Geometry check sheet. Reference: drawing and pictorial views, mm from the part's lowest x, y, z. A direction names the side the tool comes from. Round coordinates to 2 decimals unless told otherwise and drop trailing zeros. Write each loop counter-clockwise with the first axis right and the second up, starting at its lowest first coordinate (ties: lowest second). Pieces come first, ordered by that corner, then holes. Notation, with made-up numbers: M 69,14.5 L 96,14.5 A30 cw 96,53.5 Z; hole C 86.5,-40 d10. An arc over 180 degrees is marked long. Answer in a Markdown table with one row per item.
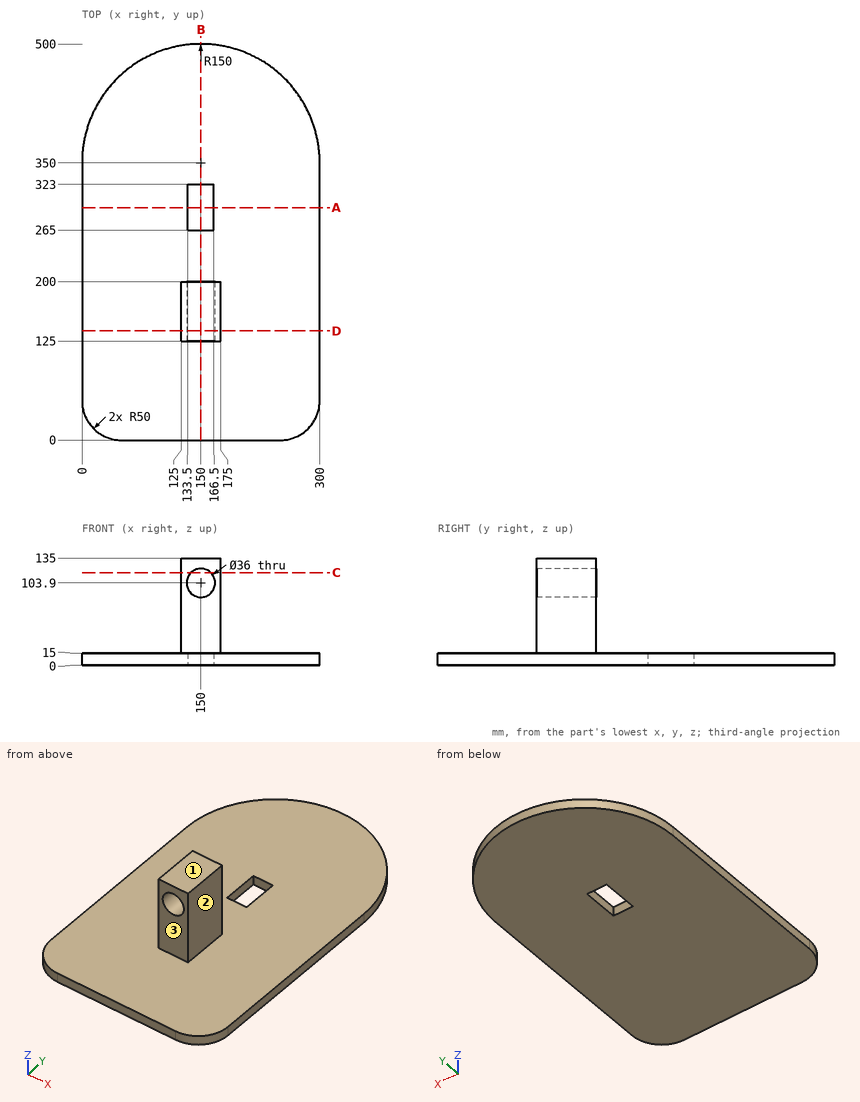
1. Section check C-C, the plane z = 117. Record the cut outline in (x, y).
Found:
| item | result |
|---|---|
| outline | M 125,125 L 137.66,125 L 137.66,200 L 125,200 Z; M 162.34,125 L 175,125 L 175,200 L 162.34,200 Z |
2. Section check B-B, the plane x = 150. Record the cut outline in (y, z).
Found:
| item | result |
|---|---|
| outline | M 0,0 L 265,0 L 265,15 L 200,15 L 200,85.9 L 125,85.9 L 125,15 L 0,15 Z; M 125,121.9 L 200,121.9 L 200,135 L 125,135 Z; M 323,0 L 500,0 L 500,15 L 323,15 Z |
3. Scan lines: L1, parallel to X at y = 154, z = 103; L2, parallel to Z at x = 150, y = 161; L3, parallel to Z at x = 220, y = 122.5. Record each from-to range of solid material in increasing order.
Found:
| item | result |
|---|---|
| L1 | x = 125 to 132.02, 167.98 to 175 |
| L2 | z = 0 to 85.9, 121.9 to 135 |
| L3 | z = 0 to 15 |
4. Section check A-A, the plane y = 293.5. Record the cut outline in (x, z), and give its area (4 significant figures).
Found:
| item | result |
|---|---|
| outline | M 0,0 L 133.5,0 L 133.5,15 L 0,15 Z; M 166.5,0 L 300,0 L 300,15 L 166.5,15 Z |
| area | 4,005 mm2 |
5. Go/stop test with flat-tipped pins: pin 1 (8 mm diameter, centred on y = 144.5, z = 92.5, fed in from +X); pin 2 (22.5 mm diameter, centred on y = 151, z = 88, fed in from -X); pin 3 (25 mm diameter, centred on x = 154, z = 73, fed in from +Y). Record where each tip stops, or that it passes through.
Found:
| item | result |
|---|---|
| pin 1 | stops at x = 175 |
| pin 2 | stops at x = 125 |
| pin 3 | stops at y = 200 |
6. Section check D-D, the plane y = 138. Record the cut outline in (x, z).
Found:
| item | result |
|---|---|
| outline | M 0,0 L 300,0 L 300,15 L 175,15 L 175,135 L 125,135 L 125,15 L 0,15 Z; hole C 150,103.9 d36 |
7. Access from +Z, -Z, +X, -X, +Y, -Y to the whole of each face (thin tool, end or side, straight path). Record for the marked faces 1, 2 and 3.
Found:
| item | result |
|---|---|
| face 1 | +Z, +X, -X, +Y, -Y |
| face 2 | +Z, +X, +Y, -Y |
| face 3 | +Z, +X, -X, -Y |
